Design review of the part built by this model. Coordinates are the model's own, in mm. Coordinates: 2 decimals unless noted, no trailing zeros. Write each loop counter-clockwise with the first axis right and the second up, starting at its lowest first coordinate (ties: lowest second). Pieces come first, ordered by that corner, then holes.
Q1. For L1, parallel to Y at x = -197, z = -0.6; L2, parallel to X at y = -33.5, z = -0.85; L3, parallel to Y at x = -215, z = -0.5, list the stretches that pass through material, from the lowest coordinate up.
Q2. Take a section at D-D, the plane x = -249.5. Write out the cut boundary in (y, z).
Q3. Take a section at B-B, the plane y = -35. Write out the cut boundary in (x, z).
Q4. Take a section at C-C, the plane z = -0.8. Write out the cut boundary in (x, y), plus the area to 3 significant figures.
Q5. Take a section at A-A, the plane x = -8. Write out the cut boundary in (y, z), plus the area to 3 significant figures.
Q6. For pin 1 Ø6.5 at (x, y) = (-8, -35) entering from +Z; pin 2 Ø0.5 at (x, z) = (-261, -0.5) entering from -Y; pin 3 Ø4 at (x, y) = (-197, -35) entering from +Z, all flat-tipped, find the tip position at first contact; note any pin that passes through.
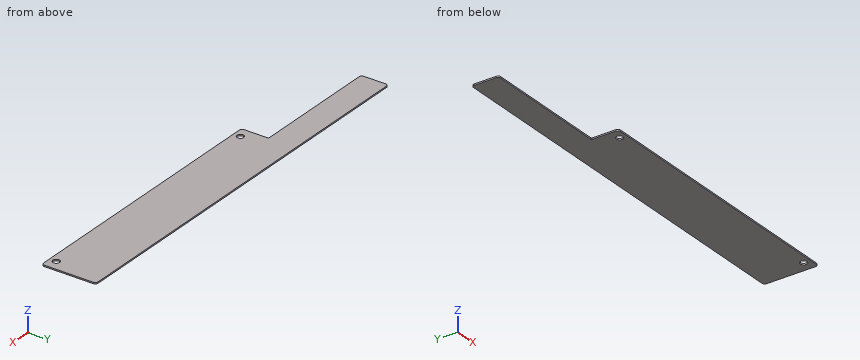
from build123d import *

# Parameters (mm, degrees)
F1_DEPTH = 1
F2_R     = 2
F3_R     = 0.5
F5_D     = 5


with BuildPart() as f1:
    # F0 (on Top) → F1 (new body)
    with BuildSketch(Plane.XY):
        Polygon((0, -40), (0, 0), (-300, 0), (-300, -20), (-205, -20), (-205, -40), align=None)
    extrude(amount=-F1_DEPTH)

    # F2
    f2_edges = [f1.edges().sort_by_distance(p)[0] for p in [
        (-300, -20, -0.5),
        (-300, 0, -0.5),
        (-205, -40, -0.5),
        (0, 0, -0.5),
        (0, -40, -0.5),
    ]]
    fillet(f2_edges, radius=F2_R)

    # F3
    f3_edges = [f1.edges().sort_by_distance(p)[0] for p in [
        (-205, -20, -0.5),
    ]]
    fillet(f3_edges, radius=F3_R)

    # F5 (through all)
    with Locations(Plane.XY):
        with Locations((-197, -35), (-8, -35)):
            Hole(F5_D / 2)


solid = f1.part
Responses:
1. L1: y = -40 to -37.5, -32.5 to 0
1. L2: x = -205 to -199, -195 to -10, -6 to 0
1. L3: y = -20 to 0
2. outline: (-20, -1) - (0, -1) - (0, 0) - (-20, 0) - close
3. outline: (-205, -1) - (-199.5, -1) - (-199.5, 0) - (-205, 0) - close; (-194.5, -1) - (-10.5, -1) - (-10.5, 0) - (-194.5, 0) - close; (-5.5, -1) - (0, -1) - (0, 0) - (-5.5, 0) - close
4. outline: (-300, -18) arc R2 ccw to (-298, -20) - (-205.5, -20) arc R0.5 cw to (-205, -20.5) - (-205, -38) arc R2 ccw to (-203, -40) - (-2, -40) arc R2 ccw to (0, -38) - (0, -2) arc R2 ccw to (-2, 0) - (-298, 0) arc R2 ccw to (-300, -2) - close; hole circle Ø5 at (-197, -35); hole circle Ø5 at (-8, -35)
4. area: 10,100 mm2
5. outline: (-40, -1) - (-37.5, -1) - (-37.5, 0) - (-40, 0) - close; (-32.5, -1) - (0, -1) - (0, 0) - (-32.5, 0) - close
5. area: 35.0 mm2
6. pin 1: stops at z = 0
6. pin 2: stops at y = -20
6. pin 3: passes through
